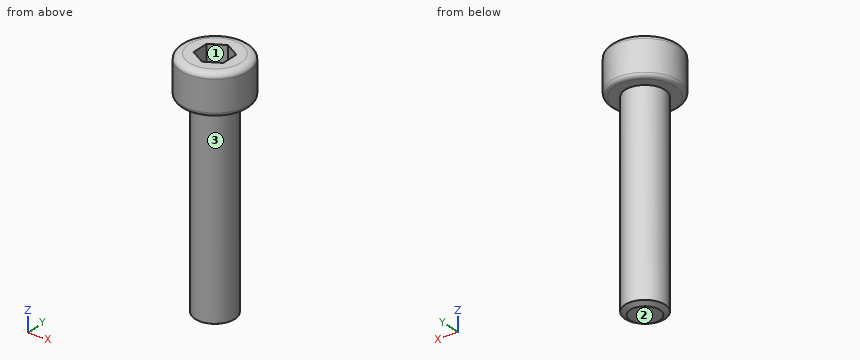
from build123d import *

# Parameters (mm, degrees)
CHAMFER_1_SIZE      = 0.3
CHAMFER_1_SIZE2     = 0.519615242
FILLET_1_R          = 0.4
FILLET_2_SIZE       = 0.5
FILLET_2_SIZE_2     = 0.8
CUT_EXTRUDE_1_DEPTH = 2


with BuildPart() as part:
    # 草图2 → 旋转1 (revolve)
    with BuildSketch(Plane(origin=(0, 0, 0), x_dir=(0, 0, -1), z_dir=(1, 0, 0)), mode=Mode.PRIVATE) as revolve_1_sk:
        Polygon((-12, 0), (-12, 3.4), (-8, 3.4), (-8, 2), (12, 2), (12, 0), align=None)
    revolve(revolve_1_sk.sketch.rotate(Axis((0, 0, -12), (0, 0, 1)), 90), axis=Axis((0, 0, -12), (0, 0, 1)))

    # 倒角1
    chamfer_1_edges = [part.edges().sort_by_distance(p)[0] for p in [
        (2, 0, -12),
    ]]
    chamfer_1_side = [part.faces().sort_by_distance(p)[0] for p in [
        (2, 0, -2),
    ]]
    chamfer(chamfer_1_edges, length=CHAMFER_1_SIZE, length2=CHAMFER_1_SIZE2, reference=chamfer_1_side[0])

    # 圆角1
    fillet_1_edges = [part.edges().sort_by_distance(p)[0] for p in [
        (3.4, 0, 8),
    ]]
    fillet(fillet_1_edges, radius=FILLET_1_R)

    # 圆角2
    # an asymmetric fillet: 0.8, 0.5 mm, written as the material it takes off along each edge
    with BuildSketch(Plane(origin=(0, 0, 12), x_dir=(-1, 0, 0), z_dir=(0, 1, 0))) as fillet_2_piece_1:
        with BuildLine():
            Bezier((3.4, -FILLET_2_SIZE), (3.4, 0), (3.4 - FILLET_2_SIZE_2, 0), weights=[1, 0.707106781, 1])
            Line((3.4 - FILLET_2_SIZE_2, 0), (3.4, 0))
            Line((3.4, 0), (3.4, -FILLET_2_SIZE))
        make_face()
    revolve(axis=Axis((0, 0, 12), (0, 0, 1)), mode=Mode.SUBTRACT)

    # 草图3 → 切除-拉伸1 (cut)
    with BuildSketch(Plane.XY.offset(12)):
        Polygon((0, 1.732050808), (-1.5, 0.866025404), (-1.5, -0.866025404), (0, -1.732050808), (1.5, -0.866025404), (1.5, 0.866025404), align=None)
    extrude(amount=-CUT_EXTRUDE_1_DEPTH, mode=Mode.SUBTRACT)


solid = part.part
Model file for the job. Use its own axes, mm. Face numbers are marked on the shaded views. Give positions to 0.01 mm unless a question says otherwise; leave off trailing zeros. Loops run counter-clockwise (first coordinate to the right, second up) from the corner with the lowest first, then second, coordinate; pieces in that order, holes last.
Item 1: Drill centre lines: line 1 along Z through (x, y) = (2.25, -0.5); line 2 along X through (y, z) = (1, -6.75); line 3 along Y through (x, z) = (0, -4.75). Where is each one in solid material? Low to high.
Check values:
line 1: z = 8 to 12
line 2: x = -1.73 to 1.73
line 3: y = -2 to 2
Item 2: Slice it at A-A (z = 4.5). Write the cut outline in (x, y), plus the area to 3 significant figures.
Check values:
outline: circle Ø4 at (0, 0)
area: 12.6 mm2
Item 3: Mould opens along X. For the marked faces 1, 2 and 3 say: +X half, -X half, draft (parallel to the pull), parting line (faces both ways), or undercut.
Check values:
face 1: undercut
face 2: draft
face 3: parting line
Item 4: Drop flat-ended pins along their axis: P1, Ø1.5, axis at y = 1.5, z = -7, coming from the +X side; P2, Ø2, axis at x = 1, z = -1, coming from the -Y side; P3, Ø4, axis at x = 2.5, z = 4, coming from the +Y side. Give the stop position or say it passes through.
Check values:
P1: stops at x = 1.85
P2: stops at y = -2
P3: stops at y = 1.94
